Part model, mm, in its own coordinate system. A direction names the side the tool comes from. Round coordinates to 2 decimals unless told otherwise and drop trailing zeros. Write each loop counter-clockwise with the first axis right and the second up, starting at its lowest first coordinate (ties: lowest second). Pieces come first, ordered by that corner, then holes. Notation, with made-up numbers: M -11,-39.5 L 1,-39.5 A26 cw 1,-0.5 Z; hole C -8.75,82 d5. An arc over 180 degrees is marked long. One line per question, with ' | ' between items. Start each with the question number.
1) Drop flat-ended pins along their axis: pin 1 Ø12 at (x, y) = (-10, 9) entering from -Z; pin 2 Ø2 at (x, z) = (1, 7.5) entering from +Y; pin 3 Ø5 at (x, z) = (-8.5, 38) entering from +Y; pin 4 Ø1.5 at (y, z) = (7, 40) entering from +X. Give the stop position or say it passes through.
2) Tool access for faces 5 (the face through (15.166, 0.087, -2.513)), 6 (the face through (-16.052, -10.487, 178.004)), 7 (the face through (16.052, -10.487, -178.004)), 8 (the face through (16.161, -10.483, 177.895)), 9 (the face through (0, -10, -180)): list every direction of +Z, -Z, +X, -X, +Y, -Y with a clear straight run to the whole face (end or side of a thin tool).
3) Saw through at B-B (y = 8). List the corners of the cut face in (x, z).
4) Saw through at A-A (z = 50.5). List the corners of the cut face in (x, y).
5) Mould opens along X. For faces 1 (the face through (0, 5, 38.9)), 2 (the face through (0, -11.243, 177)), 3 (the face through (0, -13.683, 177)), 4 (the face through (-16.161, -10.483, -177.895)) say: pulls with the +X half, pulls with the -X half, needs draft (parallel to the pull), parting line crosses it, or undercut.
6) Wall check: probe 1 along Y at (x, z) = (4, 57.5); probe 2 along Z at (x, y) = (1.5, 2.5); probe 3 along Y at (x, z) = (-11, -122.5). Give the ranges that are in metal, low to high. Write a range as [from, to].
Autodesk Inventor part; units mm, degrees
ref_plane "工作平面4" through (0, 13.6791, 0) normal (0, -1, 0) x (1, 0, 0)
ref_plane "YZ Plane" through (0, 0, 0) normal (1, 0, 0) x (0, 1, 0)
ref_plane "XZ Plane" through (0, 0, 0) normal (0, 1, 0) x (-1, 0, 0)
sketch "草圖1" plane through (0, 0, 0) normal (0, 0, 1) x (1, 0, 0)
  line L0 (-17.8, 0) -> (17.8, 0)
  line L1 (-17.8, 0) -> (17.8, 0) construction
  line L2 (-18.5, -20.4831) -> (18.5, -20.4831)
  line L3 (-17.8, 0) -> (-18.5, -20.4831)
  line L4 (17.8, 0) -> (18.5, -20.4831)
  arc A0 (17.8, 0) -> (-17.8, 0) centre (0, -499.6831) ccw
  circle A1 centre (0, 0) radius 13.6791
  line L5 (0, 13.6791) -> (0, -20.4831) construction
  line L6 (-2.1, 13.5169) -> (2.1, 13.5169)
  point P0 (0, 0)
  point P1 (0, 0)
  point P2 (-13.6785, 0.1298)
  point P3 (13.6785, 0.1298)
  point P4 (0, 0.3169)
  point P5 (0, 13.5169)
  dimension "d0" = 35.6
  dimension "d2" = 37
  dimension "d15" = 500
  dimension "d32" = 20.8
  dimension "d34" = 34
  dimension "d35" = 4.2
extrude "擠出1" add sketch "草圖1" along normal mid plane 360 contours A1 A0 L0 | A1 L0 | L0 A1 A0 | L0 L4 L2 L3 A1 | L0 A0 A1
extrude "擠出4" add sketch "草圖1" along normal mid plane 77.8 contours A0 A1 L6 | L6 A1
fillet "圓角3" radius 7 4 edges at (-18.15, -10.2415, -180) (18.15, -10.2415, -180) (18.15, -10.2415, 180) (-18.15, -10.2415, 180)
fillet "圓角4" radius 0.5 8 edges at (16.1323, 0.0566, 177.5316) (0, 0.3169, 180) (-16.1323, 0.0566, 177.5316) (-17.8, 0, 0) (-16.1323, 0.0566, -177.5316) (0, 0.3169, -180) (16.1338, 0.0566, -177.5299) (17.8, 0, 0)
sketch "草圖4" plane through (0, 0, 180) normal (0, 0, 1) x (1, 0, 0)
  line L0 (-2.94, -11.2431) -> (2.94, -11.2431)
  line L1 (2.94, -11.2431) -> (2.94, -13.6831)
  line L2 (2.94, -13.6831) -> (-2.94, -13.6831)
  line L3 (-2.94, -13.6831) -> (-2.94, -11.2431)
  circle A0 centre (2.94, -12.4631) radius 1.22
  circle A1 centre (-2.94, -12.4631) radius 1.22
  line L4 (-4.16, -12.4631) -> (4.16, -12.4631) construction
  arc A2 (10.8062, -0.3) -> (-10.8062, -0.3) centre (0, -499.6831) ccw
  line L5 (-11.4959, -20.4831) -> (11.4959, -20.4831)
  point P0 (0, 0)
  point P1 (0, -12.4631)
  point P2 (0, -0.1831)
  dimension "d28" = 2.44
  dimension "d30" = 8.32
  dimension "d31" = 6.8
ref_plane "工作平面4" through (0, 13.6791, 0) normal (0, -1, 0) x (1, 0, 0)
sketch "草圖5" plane through (0, 13.6791, 0) normal (0, -1, 0) x (1, 0, 0)
  line L0 (0, 22.28) -> (0, -22.28) construction
  line L1 (2.1, 22.28) -> (2.1, -22.28)
  line L2 (-2.1, -22.28) -> (-2.1, 22.28)
  arc A0 (2.1, 22.28) -> (-2.1, 22.28) centre (0, 22.28) ccw
  arc A1 (-2.1, -22.28) -> (2.1, -22.28) centre (0, -22.28) ccw
  line L3 (0, 24.38) -> (0, -24.38) construction
  point P0 (0, 0)
  point P1 (0, 0)
  point P2 (0, 0)
  dimension "d36" = 4.2
  dimension "d37" = 48.76
extrude "擠出6" cut sketch "草圖5" along normal blind 0.3
extrude "擠出7" cut sketch "草圖4" against normal blind 6.8
properties part number "燈"
Answer key:
1) pin 1: stops at z = -38.9 | pin 2: stops at y = 13.38 | pin 3: stops at y = 12.29 | pin 4: passes through
2) face 5: +Y | face 6: +Z, -X, +Y | face 7: -Z, +X, +Y | face 8: +Z, +X, +Y | face 9: -Z, +X, -X, +Y, -Y
3) outline: M -11.1,-38.9 L 11.1,-38.9 L 11.1,38.9 L -11.1,38.9 Z
4) outline: M -18.5,-20.48 L 18.5,-20.48 L 17.82,-0.47 A0.5 ccw 17.33,0.02 A500 ccw -17.33,0.02 A0.5 ccw -17.82,-0.47 Z
5) face 1: needs draft | face 2: undercut | face 3: undercut | face 4: pulls with the -X half
6) probe 1: y = [-20.48, 0.3] | probe 2: z = [-38.9, 38.9] | probe 3: y = [-20.48, 0.2]
